Read the model definition and answer for the solid it produces. Units are mm, in the model's axes. A direction names the side the tool comes from. Coordinates: 2 decimals unless noted, no trailing zeros. Loops run counter-clockwise (first coordinate to the right, second up) from the corner with the lowest first, then second, coordinate; pieces in that order, holes last. Notation, with made-up numbers: (10.25, -35) -> (57.25, -35) arc R11 cw to (57.25, -14) -> close; hole circle Ø4 at (89.25, 25.25). An arc over 180 degrees is marked (long way). Answer as a JSON object with one key per item and string values. Group by question number.
Q1. The part is cut by section C-C on x = -457.5. Write down the section's boundary in (y, z).
Q2. Determine the mould class of faces 1 (the flat face through (615.95, -84, 44)), 2 (the flat face through (-9, -227, 0)), 3 (the flat face through (-8, 5, 67.31)), 4 (the flat face through (558.476, -395.953, -15.936)) for opening direction Z: released by +Z, released by -Z, zero draft, split by the parting line, or undercut.
Q3. Each of these flat-tipped pins is pushed along its axis until it touches: P1, Ø5, axis at x = 65.5, y = 176, coming from the +Z side; P2, Ø6, axis at x = 197, z = 23.5, coming from the +Y side; P3, Ø12, axis at x = 213, y = 92, coming from the -Z side. Where does it stop, or does it pass through?
Q4. For faces 5 (the flat face through (-9, 356.87, 59)), 6 (the flat face through (517.91, -379.094, 56.328)), 7 (the flat face through (9, 153, 44.45)), 8 (the flat face through (-558.009, -395.953, -15.936)), determine the directions among +Z, -Z, +X, -X, +Y, -Y from which every point of the face is accessible in a straight line to the end or side of a thin tool.
Q5. The part is cut by section B-B on z = -41.5. Write down the section's boundary in (x, y) (3 decimals), and give its area (3 significant figures).
Q6. The part is cut by section A-A on y = 287.5. Write down the section's boundary in (x, z).
Q7. Straight lines are drawn through the part: line 1 along Y through (x, z) = (-496.5, 73); line 2 along X through (y, z) = (198.5, 73.5); line 3 along Z through (x, y) = (-205, 314). For each, find the intervals that lie inside material, in ascending order. Write a range as [from, to].
Q8. The part is cut by section D-D on z = 126.5. Write down the section's boundary in (x, y) (3 decimals), and give its area (3 significant figures).
from build123d import *

# Parameters (mm, degrees)
SKETCH2_W           = 1231.9
SKETCH2_H           = 713.74
BOSS_EXTRUDE1_DEPTH = 73.66
BOSS_EXTRUDE2_DEPTH = 608.33
FILLET1_R           = 12.7
CUT_EXTRUDE1_DEPTH  = 1316.517103082
CUT_EXTRUDE2_DEPTH  = 608.33
SKETCH6_W           = 1204.881325014
SKETCH6_H           = 686.721325014
CUT_EXTRUDE3_DEPTH  = 6.35


with BuildPart() as part:
    # Sketch2 → Boss-Extrude1 (new body)
    with BuildSketch(Plane.XY):
        Rectangle(SKETCH2_W, SKETCH2_H)
    extrude(amount=BOSS_EXTRUDE1_DEPTH)

    # Sketch3 → Boss-Extrude2 (add, symmetric)
    with BuildSketch(Plane(origin=(0, 0, 0), x_dir=(0, 0, -1), z_dir=(1, 0, 0))):
        Polygon((-49.53, -356.87), (-172.72, -427.99), (-153.67, -427.99), (-36.83, -369.57), (80.01, -427.99), (99.06, -427.99), (-24.13, -356.87), align=None)
    extrude(amount=BOSS_EXTRUDE2_DEPTH, both=True)

    # Fillet1
    fillet1_edges = [part.edges().sort_by_distance(p)[0] for p in [
        (0, -369.57, 36.83),
    ]]
    fillet(fillet1_edges, radius=FILLET1_R)

    # Sketch4 → Cut-Extrude1 (cut, through all)
    with BuildSketch(Plane(origin=(615.95, 0, 0), x_dir=(0, 0, -1), z_dir=(1, 0, 0))):
        Polygon((0, 356.87), (-44.45, 356.87), (-44.45, -55.88), (0, -100.33), align=None)
    extrude(amount=-CUT_EXTRUDE1_DEPTH, mode=Mode.SUBTRACT)

    # Sketch5 → Cut-Extrude2 (cut, symmetric)
    with BuildSketch(Plane.XY):
        Polygon((-608.33, -427.99), (-523.572484495, -356.87), (-608.33, -356.87), align=None)
        Polygon((-589.28, -427.99), (-485.472484495, -356.87), (485.472484495, -356.87), (589.28, -427.99), align=None)
        Polygon((608.33, -356.87), (608.33, -427.99), (523.572484495, -356.87), align=None)
    extrude(amount=CUT_EXTRUDE2_DEPTH, both=True, mode=Mode.SUBTRACT)

    # Sketch6 → Cut-Extrude3 (cut)
    with BuildSketch(Plane.XY.offset(73.66)):
        Rectangle(SKETCH6_W, SKETCH6_H)
    extrude(amount=-CUT_EXTRUDE3_DEPTH, mode=Mode.SUBTRACT)


solid = part.part
Final values:
{
 "1": {"outline": "(-356.87, 0) -> (-100.33, 0) -> (-55.88, 44.45) -> (356.87, 44.45) -> (356.87, 73.66) -> (343.36, 73.66) -> (343.36, 67.31) -> (-343.36, 67.31) -> (-343.36, 73.66) -> (-356.87, 73.66) -> close"},
 "2": {"face 1": "zero draft", "face 2": "released by -Z", "face 3": "released by +Z", "face 4": "undercut"},
 "3": {"P1": "stops at z = 67.31", "P2": "stops at y = -73.83", "P3": "stops at z = 44.45"},
 "4": {"face 5": "+Z, -Z, +X, -X, +Y", "face 6": "+Z, -Z, -Y", "face 7": "-Z, +X, -X, +Y", "face 8": "+X, -X, -Y"},
 "5": {"outline": "(-585.383, -408.735) -> (-561.175, -408.735) -> (-540.776, -394.759) -> (-568.727, -394.759) -> close; (540.776, -394.759) -> (561.175, -408.735) -> (585.383, -408.735) -> (568.727, -394.759) -> close", "area": "729 mm2"},
 "6": {"outline": "(-615.95, 44.45) -> (615.95, 44.45) -> (615.95, 73.66) -> (602.44, 73.66) -> (602.44, 67.31) -> (-602.44, 67.31) -> (-602.44, 73.66) -> (-615.95, 73.66) -> close"},
 "7": {"line 1": "y = [-356.87, -343.36], [343.36, 356.87]", "line 2": "x = [-615.95, -602.44], [602.44, 615.95]", "line 3": "z = [44.45, 67.31]"},
 "8": {"outline": "(-592.14, -414.405) -> (-569.451, -414.405) -> (-550.332, -401.306) -> (-576.53, -401.306) -> close; (550.332, -401.306) -> (569.451, -414.405) -> (592.14, -414.405) -> (576.53, -401.306) -> close", "area": "640 mm2"}
}
